Geometry: final body of the model. Coordinates: model frame, mm. Face numbers are marked on the shaded views. A direction names the side the tool comes from. Give positions to 0.01 mm unless a question says otherwise; leave off trailing zeros. Write each loop counter-clockwise with the first axis right and the second up, starting at its lowest first coordinate (ties: lowest second). Pieces come first, ordered by that corner, then holes. Notation, with made-up numbers: M -25,65.25 L 7,65.25 A19 cw 7,95.25 Z; hole C 27.5,-15.75 d10. An arc over 180 degrees is marked long. Use one line per item in the form item = value. Start each with the question number.
Item 1: Material intervals for line 1 along Z through (x, y) = (0, -39.5); line 2 along Z through (x, y) = (-30, -32); line 3 along Y through (x, z) = (-21.5, -16), sorted ascending. Write a range as from..to.
Item 2: Section query B-B on x = -30. Return loops of the section in (y, z), then the cut area to 3 significant figures.
Item 3: Pull-direction query (Y, two-part tool) for the marked faces 1, 2, 3 and 4; classes: released by +Y, released by -Y, zero draft, split by the parting line, or undercut.
Item 4: Contact query for flat-ended pins moving along their axis: P1, Ø6.5, axis at x = 0, z = 30, coming from the -Y side; P2, Ø9.5, axis at x = 0, z = 0, coming from the -Y side; P3, Ø6, axis at y = -18.5, z = -5.5, coming from the +X side; P4, Ø10, axis at y = -21.5, z = 1, coming from the -X side. Output: stop coordinate, or through.
Item 5: Section query A-A on z = 0. Return loops of the section in (x, y).
Item 6: Section query D-D on x = 0. Return loops of the section in (y, z).
Item 7: Access query for the marked faces 5 and 6. Directions: +Z, -Z, +X, -X, +Y, -Y. A direction counts if a zero-diameter tool reaches every point of the face in a straight line with its end or side. Return the directions, or none.
Item 8: Section query C-C on z = -30. Return loops of the section in (x, y).
from build123d import *

# Parameters (mm, degrees)
SKETCH_W        = 80
SKETCH_H        = 80
PAD_DEPTH       = 10
SKETCH001_W     = 40
SKETCH001_H     = 40
PAD001_DEPTH    = 20
SKETCH002_W     = 80
SKETCH002_H     = 80
PAD002_DEPTH    = 15
SKETCH003_R     = 4
POCKET_DEPTH    = 15
SKETCH004_R     = 6
POCKET001_DEPTH = 45.001


with BuildPart() as part:
    # Sketch → Pad (new body)
    with BuildSketch(Plane.XZ):
        Rectangle(SKETCH_W, SKETCH_H)
    extrude(amount=PAD_DEPTH)

    # Sketch001 (on Face6 of Pad) → Pad001 (join)
    with BuildSketch(Plane.XZ.offset(10)):
        Rectangle(SKETCH001_W, SKETCH001_H)
    extrude(amount=PAD001_DEPTH)

    # Sketch002 (on Face11 of Pad001) → Pad002 (join)
    with BuildSketch(Plane.XZ.offset(30)):
        Rectangle(SKETCH002_W, SKETCH002_H)
    extrude(amount=PAD002_DEPTH)

    # Sketch003 (on Face5 of Pad002) → Pocket (cut)
    with BuildSketch(Plane.XZ.offset(45)):
        with Locations((-30, 30)):
            Circle(SKETCH003_R)
        with Locations((30, 30)):
            Circle(SKETCH003_R)
        with Locations((30, -30)):
            Circle(SKETCH003_R)
        with Locations((-30, -30)):
            Circle(SKETCH003_R)
        with Locations((0, -30)):
            Circle(SKETCH003_R)
        with Locations((0, 30)):
            Circle(SKETCH003_R)
        with Locations((-30, 0)):
            Circle(SKETCH003_R)
        with Locations((30, 0)):
            Circle(SKETCH003_R)
    extrude(amount=-POCKET_DEPTH, mode=Mode.SUBTRACT)

    # Sketch004 (on Face5 of Pocket) → Pocket001 (cut, through all)
    with BuildSketch(Plane.XZ.offset(45)):
        Circle(SKETCH004_R)
    extrude(amount=-POCKET001_DEPTH, mode=Mode.SUBTRACT)


solid = part.part
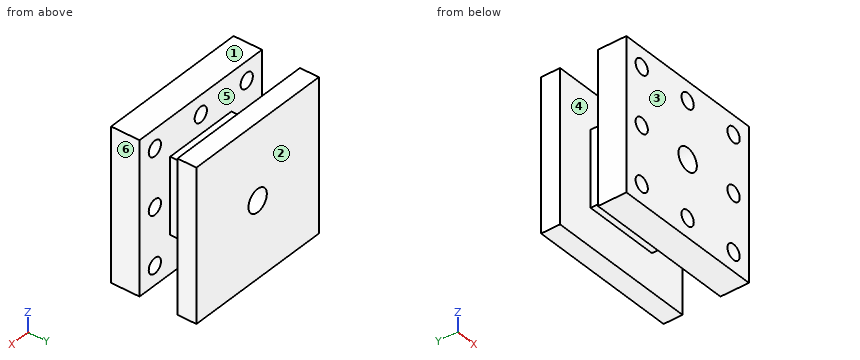
Answer sheet:
q1.line_1 = -40..-34, -26..-6, 6..26, 34..40
q1.line_2 = -40..-34, -26..-4, 4..26, 34..40
q1.line_3 = -45..-30, -10..0
q2.outline = M -45,-40 L -30,-40 L -30,-34 L -45,-34 Z; M -45,-26 L -30,-26 L -30,-4 L -45,-4 Z; M -45,4 L -30,4 L -30,26 L -45,26 Z; M -45,34 L -30,34 L -30,40 L -45,40 Z; M -10,-40 L 0,-40 L 0,40 L -10,40 Z
q2.area = 1,640 mm2
q3.face_1 = zero draft
q3.face_2 = released by +Y
q3.face_3 = released by -Y
q3.face_4 = undercut
q4.P1 = -10
q4.P2 = through
q4.P3 = 20
q4.P4 = -20
q5.outline = M -40,-45 L -34,-45 L -34,-30 L -40,-30 Z; M -40,-10 L -20,-10 L -20,-30 L -26,-30 L -26,-45 L -6,-45 L -6,0 L -40,0 Z; M 6,-45 L 26,-45 L 26,-30 L 20,-30 L 20,-10 L 40,-10 L 40,0 L 6,0 Z; M 34,-45 L 40,-45 L 40,-30 L 34,-30 Z
q6.outline = M -45,-40 L -30,-40 L -30,-34 L -45,-34 Z; M -45,-26 L -30,-26 L -30,-20 L -10,-20 L -10,-40 L 0,-40 L 0,-6 L -45,-6 Z; M -45,6 L 0,6 L 0,40 L -10,40 L -10,20 L -30,20 L -30,26 L -45,26 Z; M -45,34 L -30,34 L -30,40 L -45,40 Z
q7.face_5 = none
q7.face_6 = +Z, -Z, +X, +Y, -Y
q8.outline = M -40,-45 L -34,-45 L -34,-30 L -40,-30 Z; M -40,-10 L 40,-10 L 40,0 L -40,0 Z; M -26,-45 L -4,-45 L -4,-30 L -26,-30 Z; M 4,-45 L 26,-45 L 26,-30 L 4,-30 Z; M 34,-45 L 40,-45 L 40,-30 L 34,-30 Z
